Check sheet for the modelled part. Datum: model origin and axes. Units: mm. Round coordinates to 2 decimals unless told otherwise and drop trailing zeros. Write each loop counter-clockwise with the first axis right and the second up, starting at its lowest first coordinate (ties: lowest second). Pieces come first, ordered by that corner, then holes. Notation, with made-up numbers: (-30.75, 0.5) - (12.25, 0.5) arc R24 ccw to (12.25, 19.5) - close; hole circle Ø11 at (31, 42.5). An arc over 180 degrees is marked (long way). Use one line per item in the form item = value. Start each with the question number.
1) Gauge pin test, flat ends, axial feed: P1, Ø16.5, axis at x = -49, z = 473, coming from the +Y side; P2, Ø4, axis at y = -13, z = -84, coming from the +X side; P3, Ø5, axis at y = -17, z = 349, coming from the -X side. Record the tip position at first contact, or that the pin passes through.
2) Scan lines: probe 1 along Z at (x, y) = (0, -2.4) (3 decimals); probe 2 along X at (y, z) = (-20.5, -701.5); probe 3 along X at (y, z) = (-27, -66.5). Record each from-to range of solid material in increasing order.
3) Section check B-B (z = 423). Record the boundary of the cut face in (x, y).
4) Section check A-A (y = -16.5). Record the boundary of the cut face in (x, z).
5) Draft check along X on faces 1 (the face through (-3.9, -4.6, 1016)), 2 (the face through (0, -4.775, 14)). Enter one of: +X half, -X half, draft (parallel to the pull), parting line (faces both ways), or undercut.
Autodesk Inventor part; units mm, degrees
ref_plane "YZ Plane" through (0, 0, 0) normal (1, 0, 0) x (0, 1, 0)
ref_plane "XZ Plane" through (0, 0, 0) normal (0, 1, 0) x (-1, 0, 0)
ref_plane "XY Plane" through (0, 0, 0) normal (0, 0, 1) x (1, 0, 0)
sketch "Sketch1" plane through (0, 0, 0) normal (0, 0, 1) x (1, 0, 0)
  point P0 (0, 0)
sketch "Sketch2" plane through (0, 0, 0) normal (0, 1, 0) x (-1, 0, 0)
  line L0 (-31.75, 1016) -> (31.75, 1016)
  line L1 (31.75, 1016) -> (31.75, -1016)
  line L2 (31.75, -1016) -> (-31.75, -1016)
  line L3 (-31.75, -1016) -> (-31.75, 1016)
  line L4 (-31.75, 1016) -> (31.75, -1016) construction
  line L5 (31.75, 1016) -> (-31.75, -1016) construction
  line L6 (0, -1016) -> (0, 1016)
  point P0 (0, 0)
  point P1 (0, -657.225)
  point P2 (0, -606.425)
  point P3 (0, 657.225)
  point P4 (0, 606.425)
  point P5 (0, 0)
  dimension "d0" = 63.5
  dimension "d1" = 2032
  dimension "d24" = 50.8
  dimension "d26" = 50.8
  dimension "d27" = 1212.85
  dimension "d28" = 606.425
extrude "Plate1" add sketch "Sketch2" against normal blind 4.7752
sketch "Sketch3" plane through (36.5252, 0, 1016) normal (-1, 0, 0) x (0, -1, 0)
  line L0 (0, -2032) -> (0, 0)
  line L1 (0, 0) -> (30.1752, 0)
  line L2 (30.1752, 0) -> (30.1752, -2032)
  line L3 (30.1752, -2032) -> (0, -2032)
edge flange "Flange1" height 25.4 angle 90 thickness 4.7752 bend radius 4.7752 thickness toward (-1, 0, 0) relief tear relief width 4.7752 relief depth 2.3876 corner gap 4.7752 corner form 0 edges at (31.75, -4.7752, 0) (-31.75, -4.7752, 0) wall of the first edge with corners at (36.5252, 0, -1016) (36.5252, 0, 1016) (36.5252, -30.1752, 1016) (36.5252, -30.1752, -1016)
bend "Bend1"
corner "Corner1"
sketch "Sketch4" plane through (31.75, -34.9504, -1016) normal (0, 1, 0) x (-1, 0, 0)
  line L0 (0, 2032) -> (0, 0)
  line L1 (0, 0) -> (-30.1752, 0)
  line L2 (-30.1752, 0) -> (-30.1752, 2032)
  line L3 (-30.1752, 2032) -> (0, 2032)
edge flange "Flange2" height 25.4 angle 90 thickness 4.7752 bend radius 4.7752 thickness toward (0, 1, 0) relief tear relief width 4.7752 relief depth 2.3876 corner gap 4.7752 corner form 0 edges at (36.5252, -30.1752, 0) (-36.5252, -30.1752, 0) wall of the first edge with corners at (31.75, -34.9504, 1016) (31.75, -34.9504, -1016) (61.9252, -34.9504, -1016) (61.9252, -34.9504, 1016)
bend "Bend2"
corner "Corner2"
hole "Hole1" at (0, 0, 606.425) at (0, 0, -606.425) direction (0, -1, 0) diameter 12.7 end through all
fillet "Corner Round1" radius 6.35 4 edges at (61.9252, -32.5628, 1016) (-61.9252, -32.5628, 1016) (-61.9252, -32.5628, -1016) (61.9252, -32.5628, -1016)
equation "\"d34\" = Thickness"
equation "\"d2\" = Thickness"
equation "\"d3\" = BendReliefWidth"
equation "\"d4\" = BendReliefDepth"
equation "\"d5\" = MinimumRemnant"
equation "\"d6\" = TransitionRadius"
equation "\"d9\" = BendRadius"
equation "\"d10\" = CornerReliefSize"
equation "\"d11\" = GapSize"
equation "\"d12\" = JacobiRadiusSize"
equation "\"d13\" = BendReliefWidth"
equation "\"d14\" = BendReliefDepth"
equation "\"d15\" = MinimumRemnant"
equation "\"d16\" = TransitionRadius"
equation "\"d19\" = BendRadius"
equation "\"d20\" = CornerReliefSize"
equation "\"d21\" = GapSize"
equation "\"d22\" = JacobiRadiusSize"
equation "\"BendRadius\" = Thickness"
equation "\"BendReliefWidth\" = Thickness"
equation "\"BendReliefDepth\" = 0.5 * Thickness"
equation "\"CornerReliefSize\" = 4 * Thickness"
equation "\"MinimumRemnant\" = 2 * Thickness"
equation "\"TransitionRadius\" = BendRadius"
equation "\"JacobiRadiusSize\" = BendRadius"
equation "\"GapSize\" = Thickness"
properties part number "5th Wheel Hitch Sliding rail"
Results are:
q1.P1 = -30.14
q1.P2 = 36.53
q1.P3 = -36.53
q2.probe_1 = -1016 to -612.775, -600.075 to 600.075, 612.775 to 1016
q2.probe_2 = -36.53 to -31.75, 31.75 to 36.53
q2.probe_3 = -36.8 to -31.88, 31.88 to 36.8
q3.outline = (-61.93, -34.95) - (-41.3, -34.95) arc R9.55 ccw to (-31.75, -25.4) - (-31.75, -9.55) arc R4.78 cw to (-26.97, -4.78) - (26.97, -4.78) arc R4.78 cw to (31.75, -9.55) - (31.75, -25.4) arc R9.55 ccw to (41.3, -34.95) - (61.93, -34.95) - (61.93, -30.18) - (41.3, -30.18) arc R4.78 cw to (36.53, -25.4) - (36.53, -9.55) arc R9.55 ccw to (26.97, 0) - (-26.97, 0) arc R9.55 ccw to (-36.53, -9.55) - (-36.53, -25.4) arc R4.78 cw to (-41.3, -30.18) - (-61.93, -30.18) - close
q4.outline = (-36.53, -1016) - (-31.75, -1016) - (-31.75, 1016) - (-36.53, 1016) - close; (31.75, -1016) - (36.53, -1016) - (36.53, 1016) - (31.75, 1016) - close
q5.face_1 = draft
q5.face_2 = undercut
